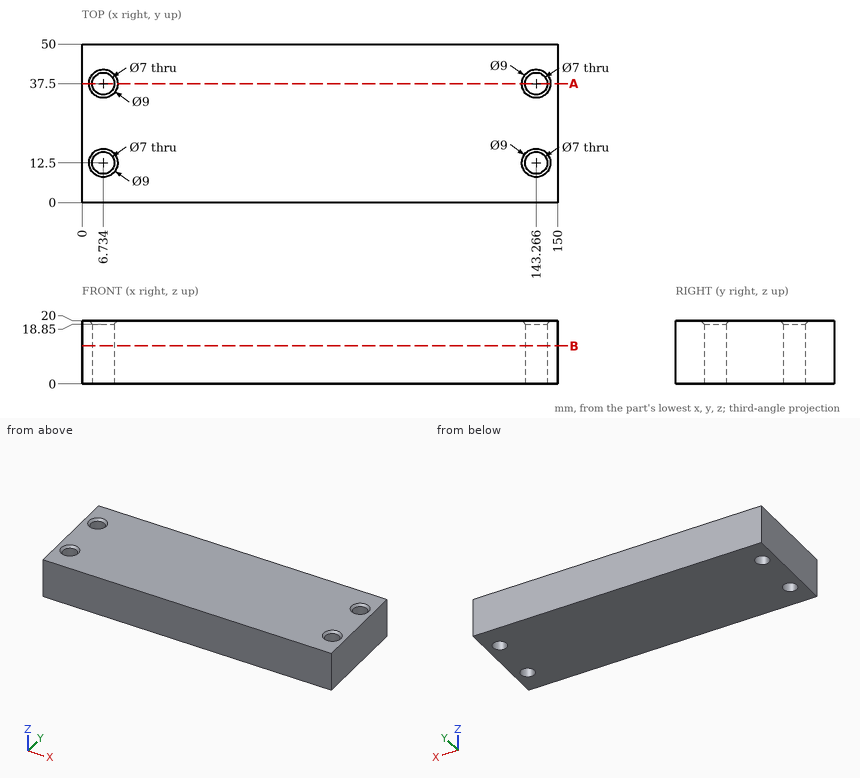
Print and shaded views of the part. All mm, measured from the part's lowest x, y and z. Round coordinates to 2 decimals unless told otherwise and drop trailing zeros. Order: outer loops, then holes, each group sorted by start corner. A loop starts at its lowest first (then second) coordinate and runs counter-clockwise, first axis right, second up.
Q1. Wall check: L1, parallel to X at y = 12.5, z = 14.5; L2, parallel to Y at x = 9.5, z = 17.75 (1 decimal); L3, parallel to X at y = 13, z = 8.25. Give the ranges that are in metal, low to high.
Q2. Drop a flat-ended pin along its axis: pin 1 (4 mm diameter, centred on x = 6.734, y = 12.5, fed in from +Z). Give the stop position or say it passes through.
Q3. Slice it at B-B (z = 12). Write the cut outline in (x, y).
Q4. Slice it at A-A (y = 37.5). Write the cut outline in (x, z).
Results below:
1. L1: x = 0 to 3.23, 10.23 to 139.77, 146.77 to 150
1. L2: y = 0 to 10.4, 14.6 to 35.4, 39.6 to 50
1. L3: x = 0 to 3.27, 10.2 to 139.8, 146.73 to 150
2. pin 1: passes through
3. outline: (0, 0) - (150, 0) - (150, 50) - (0, 50) - close; hole circle Ø7 at (6.73, 12.5); hole circle Ø7 at (6.73, 37.5); hole circle Ø7 at (143.27, 12.5); hole circle Ø7 at (143.27, 37.5)
4. outline: (0, 0) - (3.23, 0) - (3.23, 18.85) - (2.23, 20) - (0, 20) - close; (10.23, 0) - (139.77, 0) - (139.77, 18.85) - (138.77, 20) - (11.23, 20) - (10.23, 18.85) - close; (146.77, 0) - (150, 0) - (150, 20) - (147.77, 20) - (146.77, 18.85) - close
